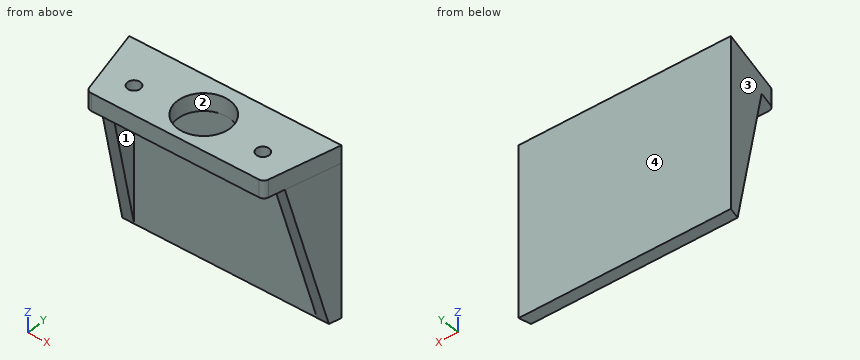
Autodesk Inventor part; units mm, degrees
ref_plane "Work Plane1" through (0, -334, 0) normal (-1, 0, 0) x (0, 0, -1)
ref_plane "YZ Plane" through (0, 0, 0) normal (1, 0, 0) x (0, 1, 0)
ref_plane "XZ Plane" through (0, 0, 0) normal (0, 1, 0) x (-1, 0, 0)
sketch "hole pattern" plane through (0, 0, 0) normal (0, 0, 1) x (1, 0, 0)
  circle A0 centre (-54.635, 0) radius 5 construction
  line L0 (-126, 0) -> (126, 0)
  line L1 (0, -37.4097) -> (0, 50.5683)
  circle A1 centre (0, 5.5) radius 22.5
  line L2 (-54.635, -5) -> (0, -5) construction
  circle A2 centre (54.635, 0) radius 5 construction
  line L3 (-90, 38) -> (90, 38)
  line L4 (-90, 38) -> (-75.9252, -20.1758)
  line L5 (-71.0654, -24) -> (71.0654, -24)
  line L6 (75.9252, -20.1758) -> (90, 38)
  circle A3 centre (-54.635, 0) radius 15 construction
  circle A4 centre (54.635, 0) radius 15 construction
  circle A5 centre (-54.635, 0) radius 5.5
  circle A6 centre (54.635, 0) radius 5.5
  arc A7 (71.0654, -24) -> (75.9252, -20.1758) centre (71.0654, -19) ccw
  arc A8 (-75.9252, -20.1758) -> (-71.0654, -24) centre (-71.0654, -19) ccw
  point P0 (0, 0)
  point P1 (-75, -24)
  point P2 (75, -24)
  dimension "d1" = 10
  dimension "d0" = 54.635
  dimension "d2" = 45
  dimension "topWidth" = 180
  dimension "d38" = 90
  dimension "d39" = 32.5
  dimension "d40" = 10.5
  dimension "d41" = 24
  dimension "d42" = 30
  dimension "d43" = 30
  dimension "d44" = 11
  dimension "d45" = 11
  dimension "d46" = 150
extrude "Extrusion1" add sketch "hole pattern" along normal blind 15 contours L4 L3 L1 A1 L0 A5 | L0 A5 A1 L1 L5 A8 L4 | L3 L6 L0 A6 A1 L1 | L1 A1 L0 A6 L6 A7 L5
sketch "Sketch2" plane through (0, 0, 0) normal (0, 0, -1) x (-1, 0, 0)
  line L0 (75.9252, -20.1758) -> (90, 38)
  line L1 (90, 38) -> (-90, 38)
  line L2 (-90, 38) -> (90, 38)
  line L3 (-90, 38) -> (90, 38)
  line L4 (-77.5806, 28) -> (77.5806, 28)
  line L5 (-69.1129, -7) -> (-77.5806, 28)
  line L6 (-69.1129, -7) -> (-79.1129, -7)
  line L7 (90, 38) -> (75.9252, -20.1758)
  line L8 (79.1129, -7) -> (69.1129, -7)
  line L9 (69.1129, -7) -> (77.5806, 28)
  line L10 (-79.1129, -7) -> (-90, 38)
  line L11 (-90, 38) -> (-75.9252, -20.1758)
  line L12 (79.1129, -7) -> (90, 38)
  point P0 (0, 0)
  dimension "d50" = 10
  dimension "d53" = 45
  dimension "d54" = 10
extrude "Extrusion2" add sketch "Sketch2" along normal blind 130
ref_plane "Work Plane1" through (0, -334, 0) normal (-1, 0, 0) x (0, 0, -1)
sketch "Sketch5" plane through (0, -334, 0) normal (-1, 0, 0) x (0, 0, -1)
  line L0 (0, -327) -> (130, -327)
  line L1 (130, -362) -> (130, -327)
  line L2 (0, -327) -> (130, -327)
  line L3 (130, -362) -> (130, -327.7477)
  line L4 (130, -362) -> (0, -327)
  point P0 (0, -334)
extrude "Extrusion3" cut sketch "Sketch5" along normal through all both and the other way through all
equation "\"d38\" = 0.5 * topWidth"
properties part number "Brake_Light_Base_Plate"
Model file for the job. Use its own axes, mm. Face numbers are marked on the shaded views. Coordinates: 2 decimals unless noted, no trailing zeros. Order: outer loops, then holes, each group sorted by start corner. A loop starts at its lowest first (then second) coordinate and runs counter-clockwise, first axis right, second up. Notation, with made-up numbers: (80.25, 45) -> (123.25, 45) arc R16 ccw to (123.25, 74) -> close; hole circle Ø6 at (26, 79.5). An arc over 180 degrees is marked (long way). Return JSON: item names as keys, results as strings. Group by question number.
Item 1: Saw through at B-B on y = 18. Write the cut outline in (x, z), then the cut area to 3 significant figures.
Item 2: Wall check: line 1 along Y through (x, z) = (0, 5); line 2 along X through (y, z) = (0, 6) (3 decimals); line 3 along Z through (x, y) = (-66, 10.5). Give the ranges that are in metal, low to high. Write a range as [from, to].
Item 3: Flat gauge pins, fed straight in: P1, Ø8, axis at x = -26, z = -37.5, coming from the -Y side; P2, Ø1.5, axis at x = -38.5, y = 12, coming from the -Z side; P3, Ø8, axis at y = 11.5, z = -39, coming from the -X side. Where does each tip first touch, or does it go through?
Item 4: Saw through at D-D on z = -66. Write the cut outline in (x, y), then the cut area to 3 significant figures.
Item 5: Saw through at A-A on x = 8.5. Write the cut outline in (y, z), then the cut area to 3 significant figures.
Item 6: Pull direction Y, two halves, no side cores. Call the marked faces 1, 2, 3 and 4: pulls with the +Y half, pulls with the -Y half, needs draft (parallel to the pull), parting line crosses it, or undercut.
Item 7: Saw through at C-C on y = 0. Write the cut outline in (x, z) (3 decimals).
Values found:
{
 "1": {"outline": "(-85.16, -92.86) -> (-75.16, -92.86) -> (-75.16, 0) -> (-18.71, 0) -> (-18.71, 15) -> (-85.16, 15) -> close; (18.71, 0) -> (75.16, 0) -> (75.16, -92.86) -> (85.16, -92.86) -> (85.16, 15) -> (18.71, 15) -> close", "area": "3,850 mm2"},
 "2": {"line 1": "y = [-24, -17], [28, 38]", "line 2": "x = [-80.806, -60.135], [-49.135, -21.817], [21.817, 49.135], [60.135, 80.806]", "line 3": "z = [0, 15]"},
 "3": {"P1": "stops at y = 28", "P2": "stops at z = 0", "P3": "stops at x = -84.56"},
 "4": {"outline": "(-90, 38) -> (-83.41, 10.77) -> (-73.41, 10.77) -> (-77.58, 28) -> (77.58, 28) -> (73.41, 10.77) -> (83.41, 10.77) -> (90, 38) -> close", "area": "2,120 mm2"},
 "5": {"outline": "(-24, 0) -> (-15.33, 0) -> (-15.33, 15) -> (-24, 15) -> close; (26.33, 0) -> (28, 0) -> (28, -130) -> (38, -130) -> (38, 15) -> (26.33, 15) -> close", "area": "1,610 mm2"},
 "6": {"face 1": "undercut", "face 2": "undercut", "face 3": "pulls with the -Y half", "face 4": "pulls with the +Y half"},
 "7": {"outline": "(-80.806, -26) -> (-70.806, -26) -> (-70.806, 0) -> (-60.135, 0) -> (-60.135, 15) -> (-80.806, 15) -> close; (-49.135, 0) -> (-21.817, 0) -> (-21.817, 15) -> (-49.135, 15) -> close; (21.817, 0) -> (49.135, 0) -> (49.135, 15) -> (21.817, 15) -> close; (60.135, 0) -> (70.806, 0) -> (70.806, -26) -> (80.806, -26) -> (80.806, 15) -> (60.135, 15) -> close"}
}
